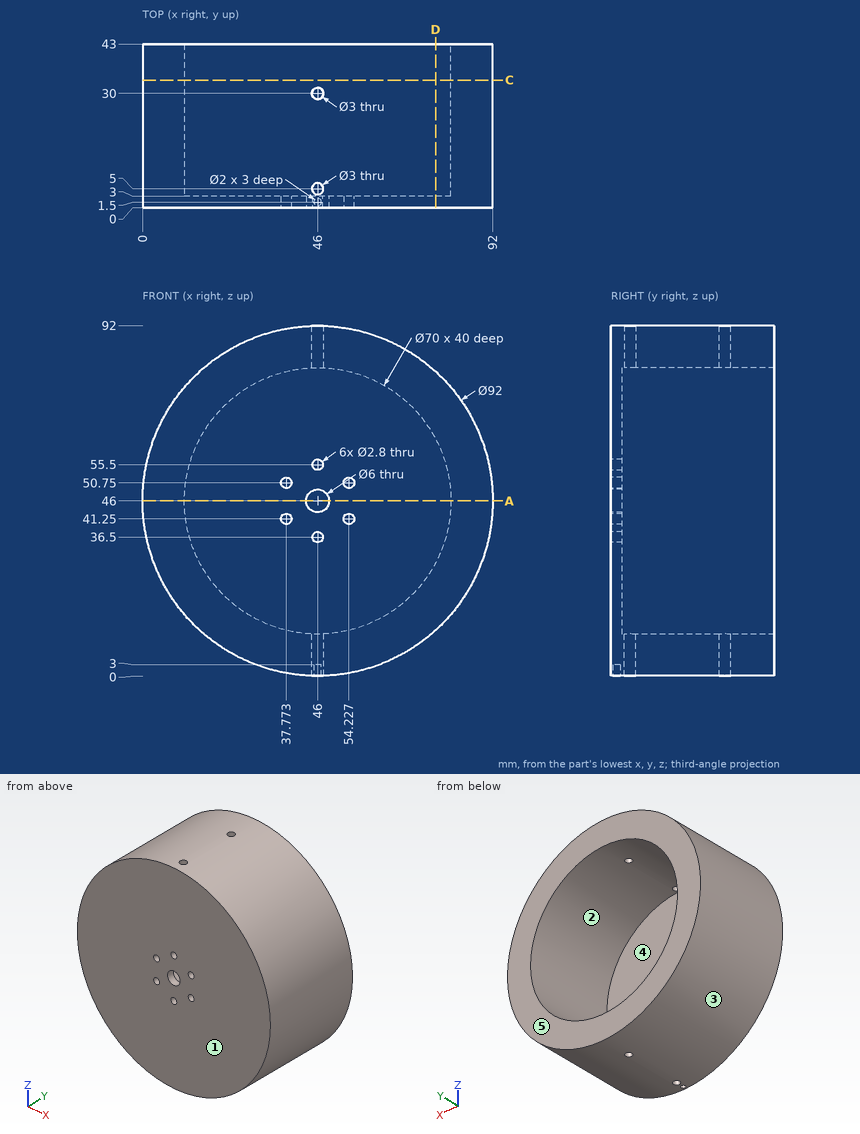
Study the drawing (mm; zero at the part's minimum x, y, z) and answer. A direction names the side the tool comes from. Round coordinates to 2 decimals unless told otherwise and drop trailing zeros. Write each loop counter-clockwise with the first axis right and the second up, starting at its lowest first coordinate (ties: lowest second). Pieces come first, ordered by that corner, then holes.
1) Flat-ended cylindrical pins translate along their axes: P1, Ø3.5, axis at x = 54.23, z = 41.25, coming from the +Y side; P2, Ø4, axis at y = 9, z = 65, coming from the +X side; P3, Ø3, axis at x = 79.5, y = 7, coming from the +Z side (1 decimal). Find the tip coordinate at first contact, or state that the pin passes through.
2) A cutting plane is placed at C-C on y = 33.5. Determine the outline of the cut face in (x, z), and give its area (3 significant figures).
3) A cutting plane is placed at A-A on z = 46. Determine the outline of the cut face in (x, y), and give its area (3 significant figures).
4) A cutting plane is placed at D-D on x = 77. Determine the outline of the cut face in (y, z) (1 decimal), and give its area (3 significant figures).
5) Determine the mould class of the marked faces 1, 2 and 3 for opening direction X: pulls with the +X half, pulls with the -X half, needs draft (parallel to the pull), parting line crosses it, or undercut.
6) Consider probe 1 along Z at (x, y) = (46, 2.1); probe 2 along Z at (x, y) = (46, 25); probe 3 along Y at (x, z) = (46, 2.5). Determine where each line is inside the solid, lowest interval first.
7) Which of the six approach directions +Z, -Z, +X, -X, +Y, -Y give full straight-line access (tool end or side, diameter ignored) to the marked faces 4 and 5?
Entries:
1. P1: stops at y = 3
1. P2: stops at x = 88.74
1. P3: stops at z = 79
2. outline: circle Ø92 at (46, 46); hole circle Ø70 at (46, 46)
2. area: 2,800 mm2
3. outline: (0, 0) - (43, 0) - (43, 3) - (11, 3) - (11, 43) - (0, 43) - close; (49, 0) - (92, 0) - (92, 43) - (81, 43) - (81, 3) - (49, 3) - close
3. area: 1,140 mm2
4. outline: (0, 12) - (43, 12) - (43, 29.8) - (3, 29.8) - (3, 62.2) - (43, 62.2) - (43, 80) - (0, 80) - close
4. area: 1,620 mm2
5. face 1: needs draft
5. face 2: undercut
5. face 3: parting line crosses it
6. probe 1: z = 3 to 35.1, 37.9 to 43, 49 to 54.1, 56.9 to 92
6. probe 2: z = 0 to 11, 81 to 92
6. probe 3: y = 0 to 0.5, 2.5 to 3.5, 6.5 to 28.5, 31.5 to 43
7. face 4: +Y
7. face 5: +Z, -Z, +X, -X, +Y
